The drawing under review shows one solid part. Ordinate dimensions are in mm from its lowest x, y, z. Give positions to 0.01 mm unless a question says otherwise; leave off trailing zeros. Loops run counter-clockwise (first coordinate to the right, second up) from the corner with the lowest first, then second, coordinate; pieces in that order, holes last. Notation, with made-up numbers: (-23, 74.25) -> (-14, 74.25) arc R14 ccw to (-14, 94.25) -> close; hole circle Ø9 at (49.25, 9). An arc over 180 degrees is marked (long way). Answer in a Markdown table with one row per item. Add a question column.
(1) Consider section B-B on y = 132.5. Write out the cut boundary in (x, z), then the cut area to 3 significant figures.
(2) Consider section A-A on x = 46. Write out the cut boundary in (y, z), then the cut area to 3 significant figures.
(3) For line 1 (Y direction, x = 52.5, z = 0.85); line 2 (X direction, y = 17.5, z = 0.75) (1 decimal); line 3 (X direction, y = 119, z = 1.95), list the stretches that pass through material, from the lowest coordinate up.
(4) Consider section C-C on z = 1.7. Write out the cut boundary in (x, y) (1 decimal).
(5) For pin 1 (0.6 mm diameter, centred on x = 82.5, z = 0.5, fed in from -Y); pin 2 (1 mm diameter, centred on x = 82.5, z = 1.5, fed in from +Y); pin 3 (0.6 mm diameter, centred on y = 73, z = 1.5, fed in from +X), all flat-tipped, find the tip position at first contact; note any pin that passes through.
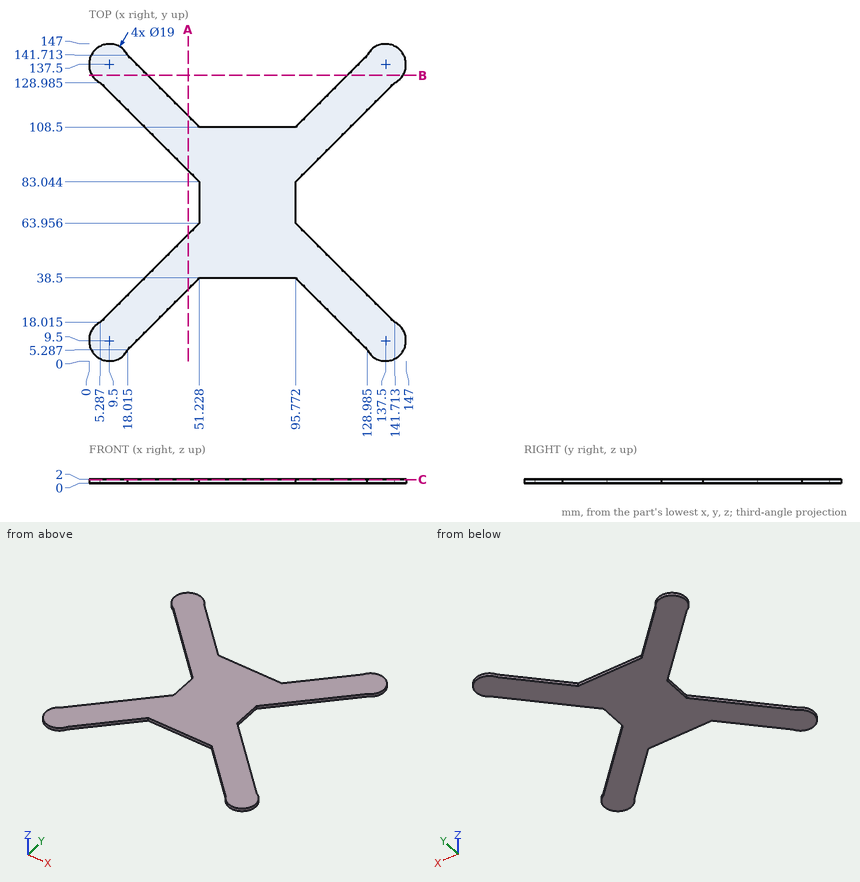
Values follow:
| question | item | result |
|---|---|---|
| 1 | outline | (1.42, 0) -> (27.23, 0) -> (27.23, 2) -> (1.42, 2) -> close; (119.77, 0) -> (145.58, 0) -> (145.58, 2) -> (119.77, 2) -> close |
| 1 | area | 103 mm2 |
| 2 | outline | (33.27, 0) -> (58.73, 0) -> (58.73, 2) -> (33.27, 2) -> close; (88.27, 0) -> (113.73, 0) -> (113.73, 2) -> (88.27, 2) -> close |
| 2 | area | 102 mm2 |
| 3 | line 1 | 38.5 to 108.5 |
| 3 | line 2 | 4.4 to 30.2, 116.8 to 142.6 |
| 3 | line 3 | 15.27 to 40.73, 106.27 to 131.73 |
| 4 | outline | (5.3, 18) arc R9.5 ccw (long way) to (18, 5.3) -> (51.2, 38.5) -> (95.8, 38.5) -> (129, 5.3) arc R9.5 ccw (long way) to (141.7, 18) -> (95.8, 64) -> (95.8, 83) -> (141.7, 129) arc R9.5 ccw (long way) to (129, 141.7) -> (95.8, 108.5) -> (51.2, 108.5) -> (18, 141.7) arc R9.5 ccw (long way) to (5.3, 129) -> (51.2, 83) -> (51.2, 64) -> close |
| 5 | pin 1 | y = 38.5 |
| 5 | pin 2 | y = 108.5 |
| 5 | pin 3 | x = 95.77 |
